```python
from build123d import *

# Parameters (mm, degrees)
SKETCH_1_W          = 103.2
SKETCH_1_H          = 90.7
SKETCH_1_W_2        = 56.5
SKETCH_1_H_2        = 71.5
EXTRUDE_1_DEPTH     = 43
EXTRUDE_3_DEPTH     = 5
SKETCH_4_R          = 3.682623049
SKETCH_4_W          = 20.371137154
SKETCH_4_H          = 17.709581546
SKETCH_4_W_2        = 16.685906313
SKETCH_4_H_2        = 21.804282482
SKETCH_4_W_3        = 16.276436219
SKETCH_4_H_3        = 17.19774393
SKETCH_4_W_4        = 16.993008883
CUT_EXTRUDE_2_DEPTH = 4.377522815
SKETCH_5_W          = 4.606538552
SKETCH_5_H          = 28.355803979
CUT_EXTRUDE_3_DEPTH = 4.922477185
SKETCH_7_R          = 1.6
CUT_EXTRUDE_4_DEPTH = 237.535409611
SKETCH_8_W          = 15
SKETCH_8_H          = 15
CUT_EXTRUDE_5_DEPTH = 15


with BuildPart() as part:
    # 草图1 → 凸台-拉伸1 (new body)
    with BuildSketch(Plane.XY):
        with BuildLine():
            Line((0, 10), (0, 39.186569494))
            ThreePointArc((0, 39.186569494), (1.375838219, 44.248568464), (5.124766715, 47.917669105))
            Line((5.124766715, 47.917669105), (10, 50.639880584))
            Line((10, 50.639880584), (10, 90))
            ThreePointArc((10, 90), (12.928932188, 97.071067812), (20, 100))
            Line((20, 100), (190, 100))
            ThreePointArc((190, 100), (197.071067812, 97.071067812), (200, 90))
            Line((200, 90), (200, 51.963395008))
            Line((200, 51.963395008), (205.683304945, 48.037782396))
            ThreePointArc((205.683304945, 48.037782396), (208.855310538, 44.455580593), (210, 39.809778695))
            Line((210, 39.809778695), (210, 10))
            ThreePointArc((210, 10), (207.071067812, 2.928932188), (200, 0))
            Line((200, 0), (10, 0))
            ThreePointArc((10, 0), (2.928932188, 2.928932188), (0, 10))
        make_face()
        with Locations((72.614593403, 50.272477185)):
            Rectangle(SKETCH_1_W, SKETCH_1_H, mode=Mode.SUBTRACT)
        with Locations((161.079111209, 50.675353005)):
            Rectangle(SKETCH_1_W_2, SKETCH_1_H_2, mode=Mode.SUBTRACT)
    extrude(amount=EXTRUDE_1_DEPTH)

    # 草图3 → 凸台-拉伸3 (add)
    with BuildSketch(Plane.XY):
        with BuildLine():
            Line((0, 10), (0, 39.186569494))
            ThreePointArc((0, 39.186569494), (1.375838219, 44.248568464), (5.124766715, 47.917669105))
            Line((5.124766715, 47.917669105), (10, 50.639880584))
            Line((10, 50.639880584), (10, 90))
            ThreePointArc((10, 90), (12.928932188, 97.071067812), (20, 100))
            Line((20, 100), (180, 100))
            ThreePointArc((180, 100), (187.071067812, 97.071067812), (190, 90))
            Line((190, 90), (190, 51.963395008))
            Line((190, 51.963395008), (195.683304945, 48.037782396))
            ThreePointArc((195.683304945, 48.037782396), (198.855310538, 44.455580593), (200, 39.809778695))
            Line((200, 39.809778695), (200, 10))
            ThreePointArc((200, 10), (197.071067812, 2.928932188), (190, 0))
            Line((190, 0), (10, 0))
            ThreePointArc((10, 0), (2.928932188, 2.928932188), (0, 10))
        make_face()
    extrude(amount=EXTRUDE_3_DEPTH)

    # 草图4 → 切除-拉伸2 (cut)
    with BuildSketch(Plane(origin=(0, 100, 0), x_dir=(1, 0, 0), z_dir=(0, 1, 0))):
        with Locations(Location((113.563696849, -10.32262821, 0), (0, 0, 180))):
            Circle(SKETCH_4_R)
        with Locations((141.053854619, -16.426982565)):
            Rectangle(SKETCH_4_W, SKETCH_4_H)
        with Locations((39.603161201, -18.474333033)):
            Rectangle(SKETCH_4_W_2, SKETCH_4_H_2)
        with Locations((67.958965179, -14.942653476)):
            Rectangle(SKETCH_4_W_3, SKETCH_4_H_3)
        with Locations((95.751747779, -14.942653476)):
            Rectangle(SKETCH_4_W_4, SKETCH_4_H_3)
    extrude(amount=-CUT_EXTRUDE_2_DEPTH, mode=Mode.SUBTRACT)

    # 草图5 → 切除-拉伸3 (cut)
    with BuildSketch(Plane.XZ):
        with Locations((34.452767739, 20.30710257)):
            Rectangle(SKETCH_5_W, SKETCH_5_H)
        with Locations((24.452767739, 20.30710257)):
            Rectangle(SKETCH_5_W, SKETCH_5_H)
        with Locations((44.452767739, 20.30710257)):
            Rectangle(SKETCH_5_W, SKETCH_5_H)
        with Locations((54.452767739, 20.30710257)):
            Rectangle(SKETCH_5_W, SKETCH_5_H)
        with Locations((64.452767739, 20.30710257)):
            Rectangle(SKETCH_5_W, SKETCH_5_H)
        with Locations((74.452767739, 20.30710257)):
            Rectangle(SKETCH_5_W, SKETCH_5_H)
        with Locations((84.452767739, 20.30710257)):
            Rectangle(SKETCH_5_W, SKETCH_5_H)
        with Locations((94.452767739, 20.30710257)):
            Rectangle(SKETCH_5_W, SKETCH_5_H)
    extrude(amount=-CUT_EXTRUDE_3_DEPTH, mode=Mode.SUBTRACT)

    # 草图7 → 切除-拉伸4 (cut, through all)
    with BuildSketch(Plane.XY.offset(43)):
        with Locations((6, 30)):
            Circle(SKETCH_7_R)
        with Locations((16, 30)):
            Circle(SKETCH_7_R)
        with Locations((16, 20)):
            Circle(SKETCH_7_R)
        with Locations((6, 20)):
            Circle(SKETCH_7_R)
        with Locations((194, 30)):
            Circle(SKETCH_7_R)
        with Locations((204, 30)):
            Circle(SKETCH_7_R)
        with Locations((204, 20)):
            Circle(SKETCH_7_R)
        with Locations((194, 20)):
            Circle(SKETCH_7_R)
    extrude(amount=-CUT_EXTRUDE_4_DEPTH, mode=Mode.SUBTRACT)

    # 草图8 → 切除-拉伸5 (cut)
    with BuildSketch(Plane.ZY):
        with Locations((35.5, 17.5)):
            Rectangle(SKETCH_8_W, SKETCH_8_H)
    cut_extrude_5 = extrude(amount=-CUT_EXTRUDE_5_DEPTH, mode=Mode.SUBTRACT)

    # 镜向1: 切除-拉伸5 across plane
    add(cut_extrude_5.mirror(Plane.ZY.offset(-105)), mode=Mode.SUBTRACT)


solid = part.part
```
Input: part model. Units: mm. Frame: model coordinates. A direction names the side the tool comes from. Round coordinates to 2 decimals unless told otherwise and drop trailing zeros. Loops run counter-clockwise (first coordinate to the right, second up) from the corner with the lowest first, then second, coordinate; pieces in that order, holes last.
1) Pin query (flat end, axial travel): pin 1 (5 mm diameter, centred on x = 6, y = 20, fed in from -Z); pin 2 (2.5 mm diameter, centred on y = 2.5, z = 25.5, fed in from -X); pin 3 (2 mm diameter, centred on y = 98, z = 14, fed in from -X); pin 4 (5.5 mm diameter, centred on y = 2.5, z = 22.5, fed in from -X). Return the tip coordinate at first contact, or that it passes through.
Ans:
pin 1: stops at z = 0
pin 2: stops at x = 2.19
pin 3: stops at x = 12.86
pin 4: stops at x = 1.2
2) Material intervals for line 1 (X direction, y = 53, z = 41.5); line 2 (X direction, y = 26, z = 21); line 3 (Y direction, x = 167.5, z = 11), sorted ascending.
Ans:
line 1: x = 10 to 21.01, 124.21 to 132.83, 189.33 to 200
line 2: x = 0 to 21.01, 124.21 to 132.83, 189.33 to 210
line 3: y = 0 to 14.93, 86.43 to 100
3) Set-up query: faces 1 (the flat face through (82.149, 2, 20)), 2 (the flat face through (7, 17, 28)), 3 (the flat face through (47.946, 98, 19)), 4 (the flat face through (161, 86.425, 24)). Return all of +Z, -Z, +X, -X, +Y, -Y with unobstructed straight access to the full face (end or side cutting, diameter ignored); none if empty.
Ans:
face 1: -Y
face 2: +Z, -X
face 3: +Y
face 4: +Z
4) Section query A-A on x = 40. Return the cut outline in (y, z), plus the area to 3 significant figures.
Ans:
outline: (0, 0) - (100, 0) - (100, 7.57) - (95.62, 7.57) - (95.62, 5) - (4.92, 5) - (4.92, 43) - (0, 43) - close; (95.62, 29.38) - (100, 29.38) - (100, 43) - (95.62, 43) - close
area: 758 mm2
5) Pull-direction query (X, two-part tool) for faces 5 (the flat face through (74, 2, 34.485)), 6 (the flat face through (195, 14, 35)), 7 (the flat face through (10, 70, 21)), 8 (the flat face through (44, 2, 6.129)); classes: released by +X, released by -X, zero draft, split by the parting line, or undercut.
Ans:
face 5: undercut
face 6: released by +X
face 7: released by -X
face 8: undercut
6) Section query B-B on z = 18.5. Count the separate pieces of the cut face and the enclosed holes in it, plus the area to 3 significant figures.
Ans:
separate pieces: 11
enclosed holes: 9
area: 5,910 mm2
7) Section query D-D on x = 157. Return the cut outline in (y, z), plus the area to 3 significant figures.
Ans:
outline: (0, 0) - (100, 0) - (100, 43) - (86.43, 43) - (86.43, 5) - (14.93, 5) - (14.93, 43) - (0, 43) - close
area: 1,580 mm2
